Could you check a few things on this model? Use its own coordinates, in mm. A direction names the side the tool comes from. Coordinates: 2 decimals unless noted, no trailing zeros. Loops run counter-clockwise (first coordinate to the right, second up) from the corner with the lowest first, then second, coordinate; pieces in that order, holes last.
from build123d import *

# Parameters (mm, degrees)
F0_R     = 8
F0_R_2   = 1.5
F1_DEPTH = 4
F2_R     = 1.5
F3_DEPTH = 25
F5_DEPTH = 12.5


with BuildPart() as f1:
    # F0 (on Top) → F1 (new body)
    with BuildSketch(Plane.XY):
        with BuildLine():
            ThreePointArc((6.9474552963, -7.192556215), (9.2052852472, -3.9067535779), (10, 0))
            ThreePointArc((10, 0), (9.2052852472, 3.9067535779), (6.9474552963, 7.192556215))
            ThreePointArc((6.9474552963, 7.192556215), (-10, 0), (6.9474552963, -7.192556215))
        make_face()
        Circle(F0_R, mode=Mode.SUBTRACT)
        with BuildLine():
            ThreePointArc((6.9474552963, 7.192556215), (9.2052852472, 3.9067535779), (10, 0))
            ThreePointArc((10, 0), (9.2052852472, -3.9067535779), (6.9474552963, -7.192556215))
            add(Edge.make_bspline(
                [(6.9474552963, -7.192556215), (8.9911078661, -5.2185452451), (12.67340799, -0.8916241092), (16.5269435239, -3.4447773085), (19.9439029761, -3.4995504174)],
                knots=[0, 0, 0, 0, 0.5019027854, 1, 1, 1, 1], degree=3))
            ThreePointArc((19.9439029761, -3.4995504174), (16.5, 0), (19.9439029761, 3.4995504174))
            add(Edge.make_bspline(
                [(6.9474552963, 7.192556215), (8.9911078661, 5.2185452451), (12.67340799, 0.8916241092), (16.5269435239, 3.4447773085), (19.9439029761, 3.4995504174)],
                knots=[0, 0, 0, 0, 0.5019027854, 1, 1, 1, 1], degree=3))
        make_face()
        with BuildLine():
            ThreePointArc((23.5, 0), (22.4549603272, 2.4946281871), (19.9439029761, 3.4995504174))
            ThreePointArc((19.9439029761, 3.4995504174), (16.5, 0), (19.9439029761, -3.4995504174))
            ThreePointArc((19.9439029761, -3.4995504174), (22.4549603272, -2.4946281871), (23.5, 0))
        make_face()
        with Locations((20, 0)):
            Circle(F0_R_2, mode=Mode.SUBTRACT)
    extrude(amount=F1_DEPTH)

    # F2 (on Front) → F3 (cut)
    with BuildSketch(Plane.XZ):
        with Locations((0, 2)):
            Circle(F2_R)
    extrude(amount=-F3_DEPTH, mode=Mode.SUBTRACT)

    # F4 (on Front) → F5 (intersect, symmetric)
    with BuildSketch(Plane.XZ):
        Polygon((10, 4), (-10, 4), (-10, -3.1432664791), (24, -2.6836021327), (24, 2.5), align=None)
    extrude(amount=F5_DEPTH, both=True, mode=Mode.INTERSECT)


solid = f1.part
1) We'd pull the mould along Y, two halves only. Please class faces 3 (the cylindrical face through (23.5, -0.1, 1.4)), 4 (the cylindrical face through (-1.73, -7.81, 1.97)), 5 (the flat face through (6, -6, 4)): released by +Y, released by -Y, zero draft, split by the parting line, or undercut.
2) If I drill on L1, parallel to Y at x = -7, z = 1.1; L2, parallel to X at y = 5.5, z = 2.65; L3, parallel to Y at x = -2, z = 1.2, over which ranges is the centre line in solid material (lowest first)?
3) Imagine slicing it at A-A on x = 0. List the corners of the cut face in (y, z) for me, plus the area to 3 significant figures.
4) Imagine slicing it at D-D on y = 8.75. List the corners of the cut face in (x, z) for me.
5) For faces 1 (the cylindrical face through (-1.5, 8.91, 2.07)), 2 (the flat face through (8, 2, 0)), which set-ups out of +Z, -Z, +X, -X, +Y, -Y let a thin tool reach every point of the face, with its end or its side?
6) Will these pins go through, and if not, where does the flat tip stop? pin 1 (2 mm diameter, centred on x = 14, z = 3, fed in from -Y); pin 2 (1.5 mm diameter, centred on x = -5.5, z = 2, fed in from +Y).
7) Imagine slicing it at C-C on x = -5. List the corners of the cut face in (y, z) for me (3 decimals).
8) Imagine slicing it at B-B on y = 0. List the corners of the cut face in (x, z) for me, plus the area to 3 significant figures.
Solved:
1. face 3: split by the parting line
1. face 4: undercut
1. face 5: zero draft
2. L1: y = -7.14 to -3.87, 3.87 to 7.14
2. L2: x = -8.35 to -5.81, 5.81 to 8.65
2. L3: y = -9.8 to -7.75, 7.75 to 9.8
3. outline: (-10, 0) - (-8, 0) - (-8, 4) - (-10, 4) - close; (8, 0) - (10, 0) - (10, 0.5) - (8, 0.5) - close; (8, 3.5) - (10, 3.5) - (10, 4) - (8, 4) - close
3. area: 10.0 mm2
4. outline: (-4.84, 0) - (4.84, 0) - (4.84, 4) - (-4.84, 4) - close; hole circle Ø3 at (0, 2)
5. face 1: +Y
5. face 2: -Z, +X, -X, +Y, -Y
6. pin 1: stops at y = -2.7
6. pin 2: stops at y = 8.8
7. outline: (-8.66, 0) - (-6.245, 0) - (-6.245, 4) - (-8.66, 4) - close; (6.245, 0) - (8.66, 0) - (8.66, 4) - (6.245, 4) - close
8. outline: (-10, 0) - (-8, 0) - (-8, 4) - (-10, 4) - close; (8, 0) - (18.5, 0) - (18.5, 3.09) - (10, 4) - (8, 4) - close; (21.5, 0) - (23.5, 0) - (23.5, 2.55) - (21.5, 2.77) - close
8. area: 51.5 mm2
